Read the model definition and answer for the solid it produces. Units are mm, in the model's axes. Face numbers are marked on the shaded views. A direction names the side the tool comes from. Round coordinates to 2 decimals unless told otherwise and drop trailing zeros. Order: outer loops, then holes, each group sorted by start corner. A loop starts at its lowest first (then second) coordinate and runs counter-clockwise, first axis right, second up. Notation, with made-up numbers: (76.5, 58.5) - (84.5, 58.5) arc R22 cw to (84.5, 82.5) - close; hole circle Ø10 at (64, 76.5). An arc over 180 degrees is marked (long way). Put each result on its own line as item: value. Start each with the question number.
Q1. Section B-B on y = 0 is taken. Give the vertices of the cut face in (x, z), then the cut area to 3 significant figures.
Q2. Section C-C on z = 94 is taken. Give the vertices of the cut face in (x, y), then the cut area to 4 significant figures.
Q3. Find the intervals of material crossed by line 1 along X through (y, z) = (2.6, 105); line 2 along Z through (x, y) = (0, -2.55); line 3 along Y through (x, z) = (5, 98.5), in increasing order. Write a range as from..to.
Q4. Which of the six approach directions +Z, -Z, +X, -X, +Y, -Y give full straight-line access (tool end or side, diameter ignored) to the marked faces 1 and 2?
Q5. Each of these flat-tipped pins is pushed along its axis until it touches: pin 1 Ø0.7 at (x, y) = (-7, 2.5) entering from -Z; pin 2 Ø5.5 at (y, z) = (0.5, 96) entering from +X; pin 3 Ø2 at (x, y) = (3, 6.5) entering from +Z; pin 4 Ø3 at (x, z) = (0, 105) entering from +Y. Where does it stop, or does it pass through?
Q6. Section D-D on z = 73 is taken. Give the vertices of the cut face in (x, y).
Q7. Section A-A on x = 0 is taken. Give the vertices of the cut face in (y, z), then the cut area to 3 significant figures.
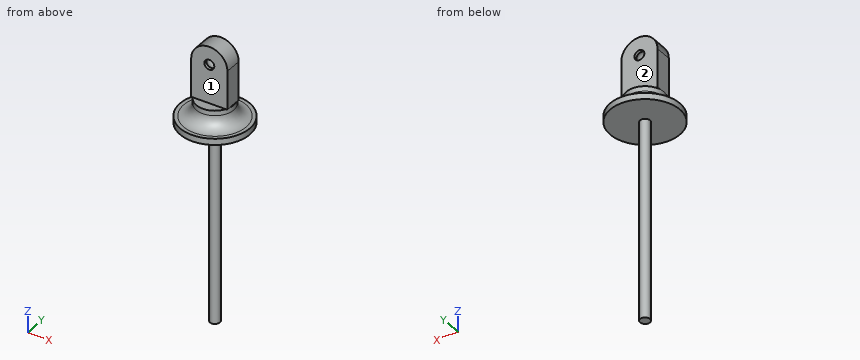
from build123d import *

# Parameters (mm, degrees)
SKETCH_1_R          = 2
EXTRUDE_1_DEPTH     = 80
SKETCH_2_R          = 14
EXTRUDE_2_DEPTH     = 2.5
SKETCH_3_R          = 7.5
EXTRUDE_3_DEPTH     = 7
FILLET_1_R          = 5
SKETCH_4_R          = 7.25
EXTRUDE_4_DEPTH     = 3.5
SKETCH_5_R          = 2
CUT_EXTRUDE_1_DEPTH = 7


with BuildPart() as part:
    # 草图1 → 凸台-拉伸1 (new body)
    with BuildSketch(Plane.XY):
        Circle(SKETCH_1_R)
    extrude(amount=EXTRUDE_1_DEPTH)

    # 草图2 → 凸台-拉伸2 (add)
    with BuildSketch(Plane.XY.offset(80)):
        Circle(SKETCH_2_R)
    extrude(amount=EXTRUDE_2_DEPTH)

    # 草图3 → 凸台-拉伸3 (add)
    with BuildSketch(Plane.XY.offset(82.5)):
        Circle(SKETCH_3_R)
    extrude(amount=EXTRUDE_3_DEPTH)

    # 圆角1
    fillet_1_edges = [part.edges().sort_by_distance(p)[0] for p in [
        (-7.5, 0, 82.5),
    ]]
    fillet(fillet_1_edges, radius=FILLET_1_R)

    # 草图4 → 凸台-拉伸4 (add, symmetric)
    with BuildSketch(Plane(origin=(0, 0, 0), x_dir=(1, 0, 0), z_dir=(0, 1, 0))):
        with BuildLine():
            ThreePointArc((-7.25, -105), (0, -97.75), (7.25, -105))
            Line((7.25, -105), (7.25, -89.5))
            Line((7.25, -89.5), (-7.25, -89.5))
            Line((-7.25, -89.5), (-7.25, -105))
        make_face()
        with Locations((0, -105)):
            Circle(SKETCH_4_R)
    extrude(amount=EXTRUDE_4_DEPTH, both=True)

    # 草图5 → 切除-拉伸1 (cut)
    with BuildSketch(Plane.XZ.offset(3.5)):
        with Locations(Location((0, 105, 0), (0, 0, 270))):
            Circle(SKETCH_5_R)
    extrude(amount=-CUT_EXTRUDE_1_DEPTH, mode=Mode.SUBTRACT)

    # 草图6 → 切除-旋转1 (revolve, cut)
    with BuildSketch(Plane(origin=(0, 0, 0), x_dir=(1, 0, 0), z_dir=(0, 1, 0))):
        with BuildLine():
            Line((0, -102), (0, -108))
            ThreePointArc((0, -108), (3, -105), (0, -102))
        make_face()
    revolve(axis=Axis((0, 0, 112.25), (0, 0, -1)), mode=Mode.SUBTRACT)


solid = part.part
Findings:
1. outline: (-14, 80) - (-2, 80) - (-2, 0) - (2, 0) - (2, 80) - (14, 80) - (14, 82.5) - (12.5, 82.5) arc R5 cw to (7.5, 87.5) - (7.5, 89.5) - (7.25, 89.5) - (7.25, 105) arc R7.25 ccw to (-7.25, 105) - (-7.25, 89.5) - (-7.5, 89.5) - (-7.5, 87.5) arc R5 cw to (-12.5, 82.5) - (-14, 82.5) - close; hole circle Ø6 at (0, 105)
1. area: 785 mm2
2. outline: (-7.25, -3.5) - (7.25, -3.5) - (7.25, 3.5) - (-7.25, 3.5) - close
2. area: 101.5 mm2
3. line 1: -7.25..-2, 2..7.25
3. line 2: 80..103, 107..112.25
3. line 3: -3.5..3.5
4. face 1: +Z, +X, -X, -Y
4. face 2: +Z, +X, -X, +Y
5. pin 1: z = 80
5. pin 2: x = 7.25
5. pin 3: z = 89.5
5. pin 4: through
6. outline: circle Ø4 at (0, 0)
7. outline: (-14, 80) - (-2, 80) - (-2, 0) - (2, 0) - (2, 80) - (14, 80) - (14, 82.5) - (12.5, 82.5) arc R5 cw to (7.5, 87.5) - (7.5, 89.5) - (3.5, 89.5) - (3.5, 103) - (2.24, 103) arc R3 cw to (-2.24, 103) - (-3.5, 103) - (-3.5, 89.5) - (-7.5, 89.5) - (-7.5, 87.5) arc R5 cw to (-12.5, 82.5) - (-14, 82.5) - close; (-3.5, 107) - (-2.24, 107) arc R3 cw to (2.24, 107) - (3.5, 107) - (3.5, 112.25) - (-3.5, 112.25) - close
7. area: 631 mm2
